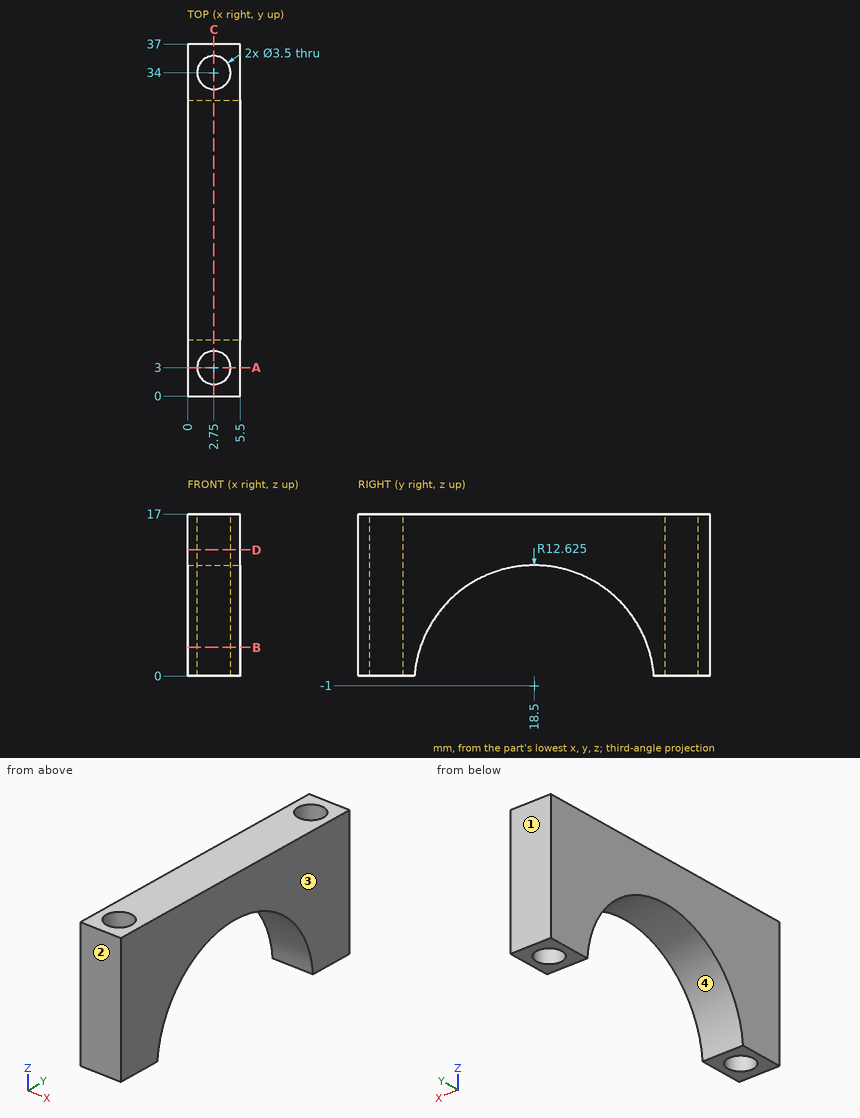
The drawing under review shows one solid part. Ordinate dimensions are in mm from its lowest x, y, z. Give positions to 0.01 mm unless a question says otherwise; leave off trailing zeros. Write each loop counter-clockwise with the first axis right and the second up, starting at its lowest first coordinate (ties: lowest second). Pieces come first, ordered by that corner, then holes. Notation, with made-up numbers: (50, 78) - (64, 78) arc R35 ccw to (64, 113) - close; hole circle Ø11 at (54, 59.25). An arc over 180 degrees is marked (long way). Answer in a Markdown table with one row per item. Add a question column.
1. Insertion check: P1, Ø3, axis at x = 2.75, y = 3, coming from the -Z side. The pin has a flat end and moves straight along its axis. Give the tip position at first contact, or say it passes through.
2. We need section C-C on x = 2.75. Write out the cut boundary in (y, z) (3 decimals).
3. Wall thickness on line 1 along X through (y, z) = (3, 8); line 2 along Y through (x, z) = (2.45, 3); line 3 along Y through (x, z) = (2.75, 3.5): over which ranges is each line inside the solid? List them lowest first. Write a range as [from, to].
4. We need section A-A on y = 3. Write out the cut boundary in (x, z), then the cut area to 3 significant figures.
5. We need section D-D on z = 13.25. Write out the cut boundary in (x, y).
6. Draft analysis for pull direction Y (two halves, no side actions). For the marked faces 1, 2, 3 and 4, state which applies: +Y half, -Y half, draft (parallel to the pull), parting line (faces both ways), or undercut.
7. We need section B-B on z = 3. Write out the cut boundary in (x, y), then the cut area to 3 significant figures.
Ans:
| question | item | result |
|---|---|---|
| 1 | P1 | passes through |
| 2 | outline | (0, 0) - (1.25, 0) - (1.25, 17) - (0, 17) - close; (4.75, 0) - (5.915, 0) arc R12.625 cw to (31.085, 0) - (32.25, 0) - (32.25, 17) - (4.75, 17) - close; (35.75, 0) - (37, 0) - (37, 17) - (35.75, 17) - close |
| 3 | line 1 | x = [0, 1], [4.5, 5.5] |
| 3 | line 2 | y = [0, 1.28], [4.72, 6.53], [30.47, 32.28], [35.72, 37] |
| 3 | line 3 | y = [0, 1.25], [4.75, 6.7], [30.3, 32.25], [35.75, 37] |
| 4 | outline | (0, 0) - (1, 0) - (1, 17) - (0, 17) - close; (4.5, 0) - (5.5, 0) - (5.5, 17) - (4.5, 17) - close |
| 4 | area | 34.0 mm^2 |
| 5 | outline | (0, 0) - (5.5, 0) - (5.5, 37) - (0, 37) - close; hole circle Ø3.5 at (2.75, 3); hole circle Ø3.5 at (2.75, 34) |
| 6 | face 1 | +Y half |
| 6 | face 2 | -Y half |
| 6 | face 3 | draft |
| 6 | face 4 | undercut |
| 7 | outline | (0, 0) - (5.5, 0) - (5.5, 6.53) - (0, 6.53) - close; (0, 30.47) - (5.5, 30.47) - (5.5, 37) - (0, 37) - close; hole circle Ø3.5 at (2.75, 3); hole circle Ø3.5 at (2.75, 34) |
| 7 | area | 52.5 mm^2 |
